Check sheet for the drawn part. Datum: minimum x, y, z corner. Units: mm. A direction names the side the tool comes from. Coordinates: 2 decimals unless noted, no trailing zeros. Loops run counter-clockwise (first coordinate to the right, second up) from the corner with the lowest first, then second, coordinate; pieces in that order, holes last. Notation, with made-up numbers: (15, -32) - (21, -32) arc R33 cw to (21, 2) - close; hole circle Ø1 at (54, 33.5). An arc over 180 degrees is marked (long way). Answer as a JSON object with one key per item and string values. Group by question number.
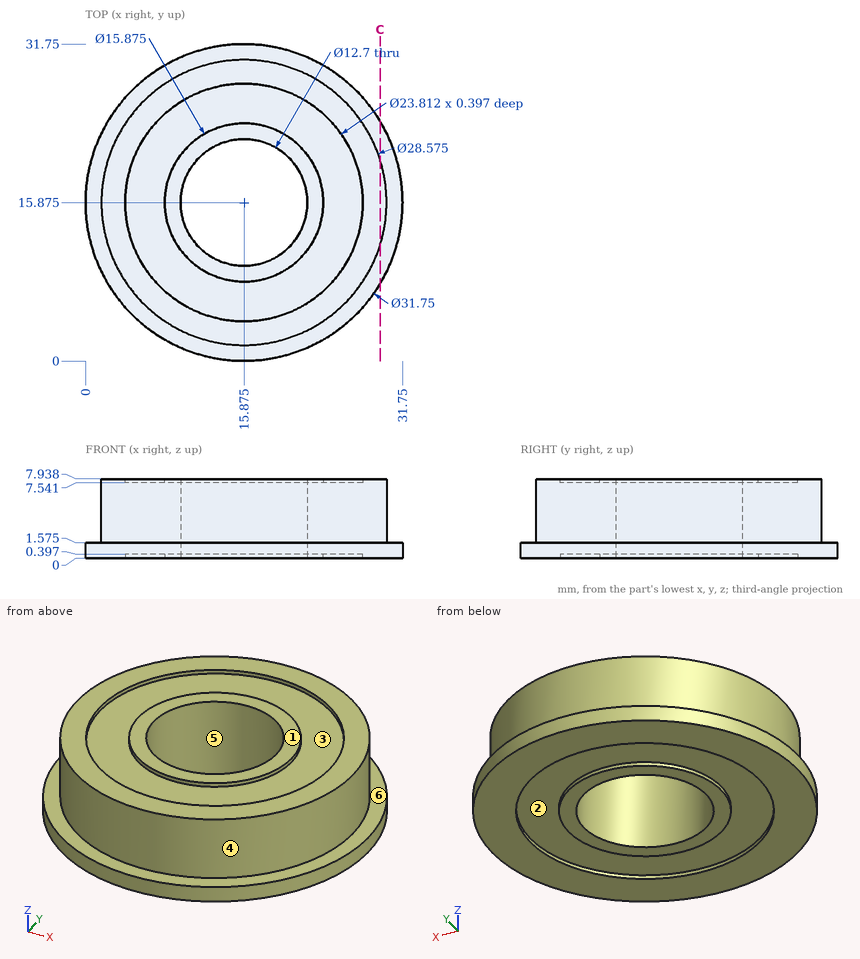
1. Sectioned sample at C-C on x = 29.5. Record the cut outline in (y, z) (1 decimal).
2. Access from +Z, -Z, +X, -X, +Y, -Y to the whole of each face (thin tool, end or side, straight path). Record for the marked faces 5 and 6.
3. Gauge pin test, flat ends, axial feed: pin 1 (4 mm diameter, centred on x = 10, z = 2.5, fed in from +Y); pin 2 (8 mm diameter, centred on x = 16.5, y = 18, fed in from -Z); pin 3 (3 mm diameter, centred on x = 25, y = 19.5, fed in from -Z); pin 4 (2 mm diameter, centred on y = 14, z = 2, fed in from +X). Record the tip position at first contact, or that the pin passes through.
4. Release check for a two-part mould opening along Y. For the marked faces 1, 2, 3 and 4 record: released by +Y, released by -Y, zero draft, split by the parting line, or undercut.
5. Material ranges on line 1 (Z direction, x = 18, y = 25); line 2 (X direction, y = 12, z = 2.5) (1 decimal); line 3 (Y direction, x = 16, z = 2.75), recorded low to high.
Answers follow:
{
 "1": {"outline": "(7.7, 0) - (24, 0) - (24, 1.6) - (20.2, 1.6) - (20.2, 7.9) - (11.6, 7.9) - (11.6, 1.6) - (7.7, 1.6) - close"},
 "2": {"face 5": "+Z, -Z", "face 6": "+Z"},
 "3": {"pin 1": "stops at y = 31.21", "pin 2": "passes through", "pin 3": "stops at z = 0.4", "pin 4": "stops at x = 31.72"},
 "4": {"face 1": "zero draft", "face 2": "undercut", "face 3": "undercut", "face 4": "split by the parting line"},
 "5": {"line 1": "z = 0.4 to 7.54", "line 2": "x = 2.1 to 10.8, 20.9 to 29.6", "line 3": "y = 1.59 to 9.53, 22.22 to 30.16"}
}
